```python
from build123d import *

# Parameters (mm, degrees)
SKETCH1_W           = 60
SKETCH1_H           = 60
BOSS_EXTRUDE1_DEPTH = 35
SKETCH2_W           = 43.4
SKETCH2_H           = 43.4
CUT_EXTRUDE1_DEPTH  = 32
SKETCH3_W           = 1.5
SKETCH3_H           = 4
CUT_EXTRUDE4_DEPTH  = 32
SKETCH7_W           = 3.5
SKETCH7_H           = 3.5
CUT_EXTRUDE7_DEPTH  = 76
BOSS_EXTRUDE4_DEPTH = 8.3
BOSS_EXTRUDE6_DEPTH = 8.3


with BuildPart() as part:
    # Sketch1 → Boss-Extrude1 (new body)
    with BuildSketch(Plane(origin=(0, 0, 0), x_dir=(1, 0, 0), z_dir=(0, 1, 0))):
        with Locations((-4.265402844, -11.303317536)):
            Rectangle(SKETCH1_W, SKETCH1_H)
    extrude(amount=BOSS_EXTRUDE1_DEPTH)

    # Sketch2 → Cut-Extrude1 (cut)
    with BuildSketch(Plane(origin=(0, 35, 0), x_dir=(1, 0, 0), z_dir=(0, 1, 0))):
        with Locations((-4.265402844, -11.303317536)):
            Rectangle(SKETCH2_W, SKETCH2_H)
    extrude(amount=-CUT_EXTRUDE1_DEPTH, mode=Mode.SUBTRACT)

    # Sketch3 → Cut-Extrude4 (cut)
    with BuildSketch(Plane(origin=(0, 3, 0), x_dir=(1, 0, 0), z_dir=(0, 1, 0))):
        with Locations((1.484597156, 12.396682464)):
            Rectangle(SKETCH3_W, SKETCH3_H)
        with Locations((1.484597156, -35.003317536)):
            Rectangle(SKETCH3_W, SKETCH3_H)
    extrude(amount=CUT_EXTRUDE4_DEPTH, mode=Mode.SUBTRACT)

    # Sketch7 → Cut-Extrude7 (cut)
    with BuildSketch(Plane.ZY.offset(34.265402844)):
        with Locations((-5.246682464, 30.75)):
            Rectangle(SKETCH7_W, SKETCH7_H)
    extrude(amount=-CUT_EXTRUDE7_DEPTH, mode=Mode.SUBTRACT)

    # Sketch9 → Boss-Extrude4 (add)
    with BuildSketch(Plane.ZY.offset(34.265402844)):
        Polygon((-6.996682464, 33.397625526), (-8.197769776, 33.397625526), (-8.197769776, 28.249822975), (-2.626030544, 28.249822975), (-2.626030544, 33.397625526), align=None)
    extrude(amount=-BOSS_EXTRUDE4_DEPTH)

    # Sketch10 → Boss-Extrude6 (add)
    with BuildSketch(Plane(origin=(25.734597156, 0, 0), x_dir=(0, 0, -1), z_dir=(1, 0, 0))):
        Polygon((3.496682464, 33.424191305), (7.449063177, 33.424191305), (7.449063177, 29.024449581), (7.449063177, 28.243284465), (2.654166816, 28.243284465), (2.654166816, 33.424191305), align=None)
    extrude(amount=-BOSS_EXTRUDE6_DEPTH)


solid = part.part
```
Here's how the part is built. I have some questions about the finished solid (model axes, mm). A direction names the side the tool comes from. Coordinates: 2 decimals unless noted, no trailing zeros. Order: outer loops, then holes, each group sorted by start corner. A loop starts at its lowest first (then second) coordinate and runs counter-clockwise, first axis right, second up. Notation, with made-up numbers: M 63,89.25 L 121,89.25 A18 cw 121,114.25 Z; hole C -20,60 d4. An arc over 180 degrees is marked long. Answer as a JSON object with one key per item and string values. Group by question number.
(1) If we mould it in two halves opening along Z, with no side actions, what happens to faces 3 (the face through (2.235, 19, -12)), 4 (the face through (25.735, 17, 12)), 5 (the face through (-5, 17, -18.697))? For each: released by +Z, released by -Z, zero draft, split by the parting line, or undercut.
(2) For pin 1 (4 mm diameter, centred on x = -20, z = 12.5, fed in from +Y), with a flat end and sliding along its axis, tell me the tip position at first contact or that it passes through.
(3) I need wall thicknesses on probe 1 along X at (y, z) = (24, 5); probe 2 along Z at (x, y) = (13, 31.5); probe 3 along X at (y, z) = (22, -12). Which ranges of each line are inside material? Lowest first, please.
(4) Which directions (+Z, -Z, +X, -X, +Y, -Y) give clear straight access to the entire face, cutting with the end or side of a thin tool? Please do faces 1 (the face through (22, 35, 11)), 2 (the face through (10, 19, -10.397)).
(5) Suppose I cut it at A-A, the plane y = 31. Please give me the cut outline in (x, z), then the cut area to 3 significant figures.
(6) Suppose I cut it at B-B, the plane z = -2.5. Please give me the cut outline in (x, y), then the cut area to 3 significant figures.
(7) Suppose I cut it at C-C, the plane x = -5. Please give me the cut outline in (y, z).
Values found:
{
 "1": {"face 3": "undercut", "face 4": "zero draft", "face 5": "released by -Z"},
 "2": {"pin 1": "stops at y = 3"},
 "3": {"probe 1": "x = -34.27 to -25.97, 17.43 to 25.73", "probe 2": "z = -18.7 to -10.4, 33 to 41.3", "probe 3": "x = -34.27 to 0.73, 2.23 to 25.73"},
 "4": {"face 1": "+Z, -Z, +X, -X, +Y", "face 2": "+Y"},
 "5": {"outline": "M -34.27,-18.7 L 25.73,-18.7 L 25.73,41.3 L -34.27,41.3 Z; hole M -25.97,-10.4 L 0.73,-10.4 L 0.73,-14.4 L 2.23,-14.4 L 2.23,-10.4 L 17.43,-10.4 L 17.43,33 L 2.23,33 L 2.23,37 L 0.73,37 L 0.73,33 L -25.97,33 Z", "area": "1,700 mm^2"},
 "6": {"outline": "M -34.27,0 L 25.73,0 L 25.73,35 L 17.43,35 L 17.43,3 L -25.97,3 L -25.97,35 L -34.27,35 Z", "area": "711 mm^2"},
 "7": {"outline": "M 0,-18.7 L 35,-18.7 L 35,-10.4 L 3,-10.4 L 3,33 L 35,33 L 35,41.3 L 0,41.3 Z"}
}
